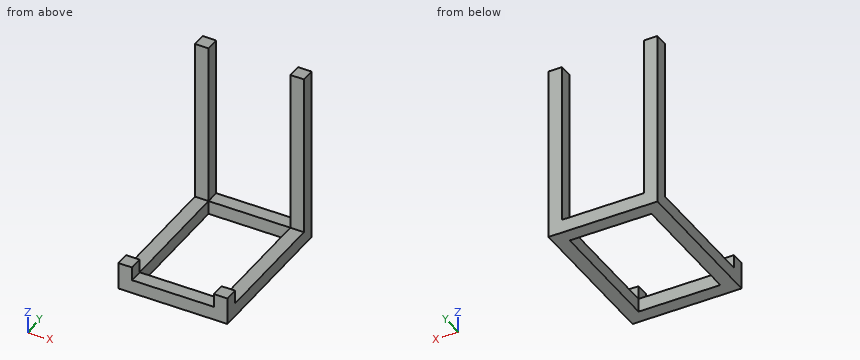
Autodesk Fusion 360 part; units mm, degrees
sketch "Sketch1" plane through (0, 0, 0) normal (0, 0, 1) x (1, 0, 0)
  line L0 (0, 0) -> (40, 0)
  line L1 (40, 0) -> (40, 55)
  line L2 (40, 55) -> (0, 55)
  line L3 (0, 55) -> (0, 0)
  line L4 (5, 5) -> (35, 5)
  line L5 (35, 5) -> (35, 50)
  line L6 (35, 50) -> (5, 50)
  line L7 (5, 50) -> (5, 5)
  dimension "d1" = 40
  dimension "d2" = 55
  dimension "d3" = 30
  dimension "d4" = 45
extrude "Extrude1" add sketch "Sketch1" along normal blind 5
sketch "Sketch2" plane through (0, 0, 5) normal (0, 0, 1) x (-1, 0, 0)
  line L0 (-5, -5) -> (-5, -50)
  line L1 (-5, -50) -> (-35, -50)
  line L2 (-35, -50) -> (-35, -5)
  line L3 (-35, -5) -> (-5, -5)
  line L4 (0, -55) -> (0, 0)
  line L5 (0, 0) -> (-40, 0)
  line L6 (-40, 0) -> (-40, -55)
  line L7 (-40, -55) -> (0, -55)
  line L8 (0, -55) -> (-5, -55)
  line L9 (-5, -55) -> (-5, -50)
  line L10 (-5, -50) -> (0, -50)
  line L11 (0, -50) -> (0, -55)
  line L12 (-35, -55) -> (-40, -55)
  line L13 (-40, -55) -> (-40, -50)
  line L14 (-40, -50) -> (-35, -50)
  line L15 (-35, -50) -> (-35, -55)
  line L16 (-35, -5) -> (-40, -5)
  line L17 (-40, -5) -> (-40, 0)
  line L18 (-40, 0) -> (-35, 0)
  line L19 (-35, 0) -> (-35, -5)
  line L20 (0, -5) -> (-5, -5)
  line L21 (-5, -5) -> (-5, 0)
  line L22 (-5, 0) -> (0, 0)
  line L23 (0, 0) -> (0, -5)
extrude "Extrude2" add sketch "Sketch2" along normal blind 5 contours L4 L5 L20 L21 L22 L23 | L5 L6 L16 L17 L18 L19
extrude "Extrude3" add sketch "Sketch2" along normal blind 60 contours L4 L7 L8 L9 L10 L11 | L6 L7 L12 L13 L14 L15
Here's how the part is built. I have some questions about the finished solid (model axes, mm). Give positions to 0.01 mm unless a question says otherwise; leave off trailing zeros. Order: outer loops, then holes, each group sorted by start corner. A loop starts at its lowest first (then second) coordinate and runs counter-clockwise, first axis right, second up. Notation, with made-up numbers: M 53.25,1 L 61.25,1 A16 ccw 61.25,30 Z; hole C 4.5,-3 d1. An arc over 180 degrees is marked long. Use a Markdown table: item, result. Add a question column.
1. Suppose I cut it at D-D (x = 3.5). List the corners of the cut face in (y, z) for me.
2. Suppose I cut it at B-B (z = 20). List the corners of the cut face in (x, y) for me.
3. I need wall thicknesses on probe 1 along Y at (x, z) = (4, 7); probe 2 along X at (y, z) = (51, 47.5); probe 3 along Z at (x, y) = (11.5, 4.5). Which ranges of each line are inside material? Lowest first, please. Write a range as from..to.
4. For pin 1 Ø2.5 at (x, z) = (2.5, 46.5) entering from -Y; pin 2 Ø2.5 at (x, y) = (2.5, 36.5) entering from +Z; pin 3 Ø8 at (y, z) = (29.5, 12) entering from -X, each with a flat end and sliding along its axis, tell me the tip position at first contact or that it passes through.
5. Suppose I cut it at A-A (y = 22). List the corners of the cut face in (x, z) for me, and give its area (3 significant figures).
6. Suppose I cut it at C-C (y = 51.5). List the corners of the cut face in (x, z) for me, and give its area (3 significant figures).
Results list:
| question | item | result |
|---|---|---|
| 1 | outline | M 0,0 L 55,0 L 55,65 L 50,65 L 50,5 L 5,5 L 5,10 L 0,10 Z |
| 2 | outline | M 0,50 L 5,50 L 5,55 L 0,55 Z; M 35,50 L 40,50 L 40,55 L 35,55 Z |
| 3 | probe 1 | y = 0..5, 50..55 |
| 3 | probe 2 | x = 0..5, 35..40 |
| 3 | probe 3 | z = 0..5 |
| 4 | pin 1 | stops at y = 50 |
| 4 | pin 2 | stops at z = 5 |
| 4 | pin 3 | passes through |
| 5 | outline | M 0,0 L 5,0 L 5,5 L 0,5 Z; M 35,0 L 40,0 L 40,5 L 35,5 Z |
| 5 | area | 50.0 mm² |
| 6 | outline | M 0,0 L 40,0 L 40,65 L 35,65 L 35,5 L 5,5 L 5,65 L 0,65 Z |
| 6 | area | 800 mm² |
